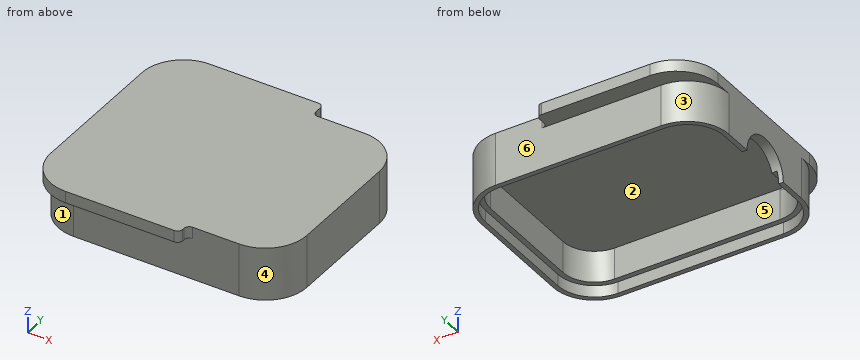
from build123d import *

# Parameters (mm, degrees)
F1_DEPTH     = 10.25
F3_DEPTH     = 2.25
F4_R         = 1
F5_T         = 1.9
F5_T3_DEPTH  = 4.8
F5_T5_DEPTH  = 25.8
F5_T8_ANGLE  = 90.000000001
F5_T10_ANGLE = 90.000000001
F7_DEPTH     = 2.25
F9_DEPTH     = 6.4


# Not quite as in the source:
# - a shell that OpenCascade refuses in one call is made with other operations: the cavity is built on its own and cut out


with BuildPart() as f1:
    # F0 (on Top) → F1 (new body)
    with BuildSketch(Plane.XY):
        with BuildLine():
            Line((16, 19), (-16, 19))
            ThreePointArc((-16, 19), (-21.6568542495, 16.6568542495), (-24, 11))
            Line((-24, 11), (-24, -11))
            ThreePointArc((-24, -11), (-21.6568542495, -16.6568542495), (-16, -19))
            Line((-16, -19), (16, -19))
            ThreePointArc((16, -19), (21.6568542495, -16.6568542495), (24, -11))
            Line((24, -11), (24, 11))
            ThreePointArc((24, 11), (21.6568542495, 16.6568542495), (16, 19))
        make_face()
    extrude(amount=F1_DEPTH)

    # F2 (on face) → F3 (join)
    with BuildSketch(Plane.XY.offset(10.25)):
        with BuildLine():
            Line((6, 22.309198174), (-16, 22.309198174))
            ThreePointArc((-16, 22.309198174), (-21.6568542495, 19.9660524235), (-24, 14.309198174))
            Line((-24, 14.309198174), (-24, 11))
            ThreePointArc((-24, 11), (-21.6568542495, 16.6568542495), (-16, 19))
            Line((-16, 19), (6, 19))
            Line((6, 19), (6, 22.309198174))
        make_face()
        with BuildLine():
            Line((6, -21.390801826), (6, -19))
            Line((6, -19), (-16, -19))
            ThreePointArc((-16, -19), (-21.6568542495, -16.6568542495), (-24, -11))
            Line((-24, -11), (-24, -13.390801826))
            ThreePointArc((-24, -13.390801826), (-21.6568542495, -19.0476560755), (-16, -21.390801826))
            Line((-16, -21.390801826), (6, -21.390801826))
        make_face()
    extrude(amount=-F3_DEPTH)

    # F4
    f4_edges = [f1.edges().sort_by_distance(p)[0] for p in [
        (6, -21.390802, 9.125),
        (6, -19, 9.125),
        (6, 19, 9.125),
        (6, 22.309198, 9.125),
    ]]
    fillet(f4_edges, radius=F4_R)

    # F5: shell of thickness 1.9, made by hand


with BuildPart() as f5_core1:
    # F5_t2: copy of F1
    add(f1.part)

    # the walls: a layer under each face that stays
    f5_faces = [f5_core1.faces().sort_by_distance(p)[0] for p in [
        (0, 19, 5.125),
        (0, 0.459198174, 10.25),
        (6.2928932188, 19.2928932188, 9.125),
        (21.6568542495, 16.6568542495, 5.125),
        (-18.8333333333, 20.4243318117, 8),
        (-21.6568542495, 16.6568542495, 4),
        (6, 20.654599087, 9.125),
        (24, 0, 5.125),
        (21.6568542495, -16.6568542495, 5.125),
        (-5.5, 22.309198174, 9.125),
        (0, -19, 5.125),
        (-21.6568542495, 19.9660524235, 9.125),
        (6.2928932188, -19.2928932188, 9.125),
        (-24, 0.459198174, 5.125),
        (6, -20.195400913, 9.125),
        (-21.6568542495, -19.0476560755, 9.125),
        (-5.5, -21.390801826, 9.125),
        (-21.6568542495, -16.6568542495, 4),
        (-18.8333333333, -19.6590015216, 8),
    ]]
    thicken(f5_faces, amount=-F5_T, mode=Mode.SUBTRACT)

    # F5_s4 → F5_t3 (cut)
    with BuildSketch(Plane.YZ.offset(4.1)):
        Polygon((19.019, 7.981), (17.1, 8), (17.1, 9.9), (19, 9.9), align=None)
        Polygon((-19.019, 7.981), (-17.1, 8), (-17.1, 9.9), (-19, 9.9), align=None)
    extrude(amount=F5_T3_DEPTH, mode=Mode.SUBTRACT)

    # F5_s6 → F5_t5 (cut)
    with BuildSketch(Plane.YZ.offset(-17.9)):
        Polygon((19.019, 7.981), (17.1, 8), (17.1, 9.9), (19, 9.9), align=None)
        Polygon((-19.019, 7.981), (-17.1, 8), (-17.1, 9.9), (-19, 9.9), align=None)
    extrude(amount=F5_T5_DEPTH, mode=Mode.SUBTRACT)

    # F5_s7 → F5_t8 (revolve, cut)
    with BuildSketch(Plane.XZ.offset(-11)):
        Polygon((-24.019, 7.981), (-24, 9.9), (-22.1, 9.9), (-22.1, 8), align=None)
    revolve(axis=Axis((-16, 11, 8), (0, 0, -1)), revolution_arc=F5_T8_ANGLE, mode=Mode.SUBTRACT)

    # F5_s9 → F5_t10 (revolve, cut)
    with BuildSketch(Plane.YZ.offset(-16)):
        Polygon((-19.019, 7.981), (-17.1, 8), (-17.1, 9.9), (-19, 9.9), align=None)
    revolve(axis=Axis((-16, -11, 8), (0, 0, -1)), revolution_arc=F5_T10_ANGLE, mode=Mode.SUBTRACT)


with BuildPart() as f1_1:
    add(f1.part)

    # what is left inside the walls is the cavity
    f5_cavity = [f5_core1.part.solids().sort_by_distance(p)[0] for p in [
        (0, -5.7, 0.019),
    ]]
    add(f5_cavity, mode=Mode.SUBTRACT)

    # F6 (on face) → F7 (cut)
    with BuildSketch(Plane(origin=(0, 0, 0), x_dir=(1, 0, 0), z_dir=(0, 0, -1))):
        with BuildLine():
            ThreePointArc((-16, 18.1000009179), (-21.0204587955, 16.0204587955), (-23.1000009179, 11))
            Line((-23.1000009179, 11), (-23.1000009179, -11))
            ThreePointArc((-23.1000009179, -11), (-21.0204587955, -16.0204587955), (-16, -18.1000009179))
            Line((-16, -18.1000009179), (16, -18.1000009179))
            ThreePointArc((16, -18.1000009179), (21.0204587955, -16.0204587955), (23.1000009179, -11))
            Line((23.1000009179, -11), (23.1000009179, 11))
            ThreePointArc((23.1000009179, 11), (21.0204587955, 16.0204587955), (16, 18.1000009179))
            Line((16, 18.1000009179), (-16, 18.1000009179))
        make_face()
        with BuildLine():
            Line((16, -17.1), (-16, -17.1))
            ThreePointArc((-16, -17.1), (-20.3133513652, -15.3133513652), (-22.1, -11))
            Line((-22.1, -11), (-22.1, 11))
            ThreePointArc((-22.1, 11), (-20.3133513652, 15.3133513652), (-16, 17.1))
            Line((-16, 17.1), (16, 17.1))
            ThreePointArc((16, 17.1), (20.3133513652, 15.3133513652), (22.1, 11))
            Line((22.1, 11), (22.1, -11))
            ThreePointArc((22.1, -11), (20.3133513652, -15.3133513652), (16, -17.1))
        make_face(mode=Mode.SUBTRACT)
    extrude(amount=-F7_DEPTH, mode=Mode.SUBTRACT)

    # F8 (on face) → F9 (cut)
    with BuildSketch(Plane(origin=(-24, 0, 0), x_dir=(0, -1, 0), z_dir=(-1, 0, 0))):
        with BuildLine():
            Line((-5.5, 0), (5.5, 0))
            ThreePointArc((5.5, 0), (0, 5.5), (-5.5, 0))
        make_face()
    extrude(amount=-F9_DEPTH, mode=Mode.SUBTRACT)


solid = f1_1.part
Work out the finished part from the listing and answer in its coordinate system (mm). Face numbers are marked on the shaded views. A direction names the side the tool comes from. Round coordinates to 2 decimals unless told otherwise and drop trailing zeros. Loops run counter-clockwise (first coordinate to the right, second up) from the corner with the lowest first, then second, coordinate; pieces in that order, holes last. Notation, with made-up numbers: M 83.25,-28 L 101.25,-28 A18 cw 101.25,1 Z; hole C 76,35 d6. An arc over 180 degrees is marked long. One line per question, with ' | ' between items. Start each with the question number.
(1) Find the intervals of material crossed by line 1 (Y direction, x = -5.5, z = 6.25); line 2 (Y direction, x = 7, z = 1.25); line 3 (X direction, y = 5, z = 6.5), in increasing order.
(2) A cutting plane is placed at C-C on y = 0. Write down the section's boundary in (x, z).
(3) A cutting plane is placed at B-B on x = -8. Write down the section's boundary in (y, z).
(4) For a pull along X with two mould halves and no side action, classify the marked faces 4, 5 and 6 as released by +X, released by -X, zero draft, split by the parting line, or undercut.
(5) A cutting plane is placed at D-D on x = 14. Write down the section's boundary in (y, z), plus the area to 3 significant figures.
(6) A tool of negligible diameter and unlimited length cuts with its end or side. For the marked faces 1, 2 and 3, from which of +Z, -Z, +X, -X, +Y, -Y can it reach the whole face along a straight path? Write none if from no direction.
(7) A cutting plane is placed at A-A on z = 6.5. Write down the section's boundary in (x, y), plus the area to 3 significant figures.
(8) Flat-ended cylindrical pins translate along their axes: pin 1 Ø3 at (x, z) = (-7, 6) entering from +Y; pin 2 Ø6 at (y, z) = (-4.5, 1.5) entering from -X; pin 3 Ø18 at (x, y) = (-8, -0.5) entering from -Z; pin 4 Ø1.4 at (y, z) = (20.5, 9.5) entering from +X. Find the tip coordinate at first contact, or state that the pin passes through.
Geometry check:
1) line 1: y = -19 to -17.1, 17.1 to 19 | line 2: y = -19 to -18.1, 18.1 to 19 | line 3: x = -24 to -22.1, 22.1 to 24
2) outline: M -24,5.5 L -22.1,5.5 L -22.1,8.35 L 22.1,8.35 L 22.1,2.25 L 23.1,2.25 L 23.1,0 L 24,0 L 24,10.25 L -24,10.25 Z
3) outline: M -21.39,8 L -19,8 L -19,0 L -18.1,0 L -18.1,2.25 L -17.1,2.25 L -17.1,8.35 L 17.1,8.35 L 17.1,2.25 L 18.1,2.25 L 18.1,0 L 19,0 L 19,8 L 22.31,8 L 22.31,10.25 L -21.39,10.25 Z
4) face 4: released by +X | face 5: undercut | face 6: zero draft
5) outline: M -19,0 L -18.1,0 L -18.1,2.25 L -17.1,2.25 L -17.1,8.35 L 17.1,8.35 L 17.1,2.25 L 18.1,2.25 L 18.1,0 L 19,0 L 19,10.25 L -19,10.25 Z | area: 99.4 mm²
6) face 1: -Z, -X, -Y | face 2: -Z | face 3: -Z, -X, +Y
7) outline: M -24,-11 A8 ccw -16,-19 L 16,-19 A8 ccw 24,-11 L 24,11 A8 ccw 16,19 L -16,19 A8 ccw -24,11 Z; hole M -22.1,-11 A6.1 ccw -16,-17.1 L 16,-17.1 A6.1 ccw 22.1,-11 L 22.1,11 A6.1 ccw 16,17.1 L -16,17.1 A6.1 ccw -22.1,11 Z | area: 289 mm²
8) pin 1: stops at y = 19 | pin 2: stops at x = -24 | pin 3: stops at z = 8.35 | pin 4: stops at x = 6.02
